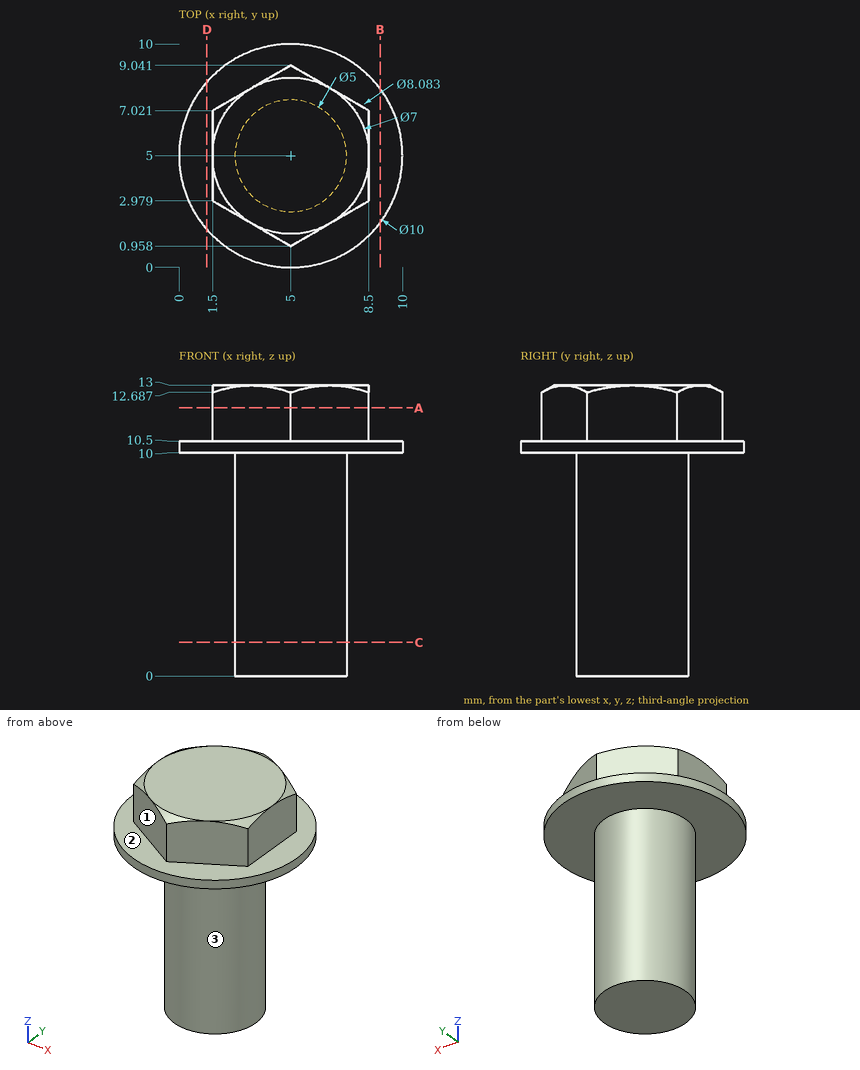
Study the drawing (mm; zero at the part's minimum x, y, z) and answer. A direction names the side the tool comes from. Give positions to 0.01 mm unless a question says otherwise; leave off trailing zeros. Write each loop counter-clockwise with the first axis right and the second up, starting at its lowest first coordinate (ties: lowest second). Pieces come first, ordered by that corner, then holes. Notation, with made-up numbers: (40.25, 24.25) -> (99.25, 24.25) arc R29 ccw to (99.25, 55.25) -> close; hole circle Ø11 at (70.5, -8.5). An arc over 180 degrees is marked (long way). Write item = value, one per line. Start each with the question number.
1) The part is cut by section D-D, the plane x = 1.25. Determine the outline of the cut face in (y, z).
2) The part is cut by section B-B, the plane x = 9. Determine the outline of the cut face in (y, z).
3) Straight lines are drawn through the part: line 1 along Z through (x, y) = (1, 4); line 2 along Y through (x, z) = (5, 6); line 3 along Z through (x, y) = (3, 7). For each, find the intervals that lie inside material, in ascending order.
4) The part is cut by section C-C, the plane z = 1.5. Determine the outline of the cut face in (x, y).
5) The part is cut by section A-A, the plane z = 12. Determine the outline of the cut face in (x, y).
6) Each of these flat-tipped pins is pushed along its axis until it touches: pin 1 (0.8 mm diameter, centred on y = 5.5, z = 11.5, fed in from -X); pin 2 (1.5 mm diameter, centred on x = 8, z = 10, fed in from -Y) (1 decimal); pin 3 (1 mm diameter, centred on y = 6.5, z = 3, fed in from -X). Where does it stop, or does it pass through?
7) Which of the six approach directions +Z, -Z, +X, -X, +Y, -Y give full straight-line access (tool end or side, diameter ignored) to the marked faces 1, 2 and 3?
Solutions:
q1.outline = (1.69, 10) -> (8.31, 10) -> (8.31, 10.5) -> (1.69, 10.5) -> close
q2.outline = (2, 10) -> (8, 10) -> (8, 10.5) -> (2, 10.5) -> close
q3.line_1 = 10 to 10.5
q3.line_2 = 2.5 to 7.5
q3.line_3 = 10 to 13
q4.outline = circle Ø5 at (5, 5)
q5.outline = (1.5, 2.98) -> (5, 0.96) -> (8.5, 2.98) -> (8.5, 7.02) -> (5, 9.04) -> (1.5, 7.02) -> close
q6.pin_1 = 1.5
q6.pin_2 = 0.5
q6.pin_3 = 2.71
q7.face_1 = +Z, -X, -Y
q7.face_2 = +Z
q7.face_3 = -Z
